Input: dimensioned drawing with shaded views. Units: mm. Origin: part minimum x, y, z. A direction names the side the tool comes from. Give positions to 0.01 mm unless a question says otherwise; leave off trailing zeros. Write each loop counter-clockwise with the first axis right and the second up, starting at its lowest first coordinate (ties: lowest second). Pieces come first, ordered by that corner, then holes.
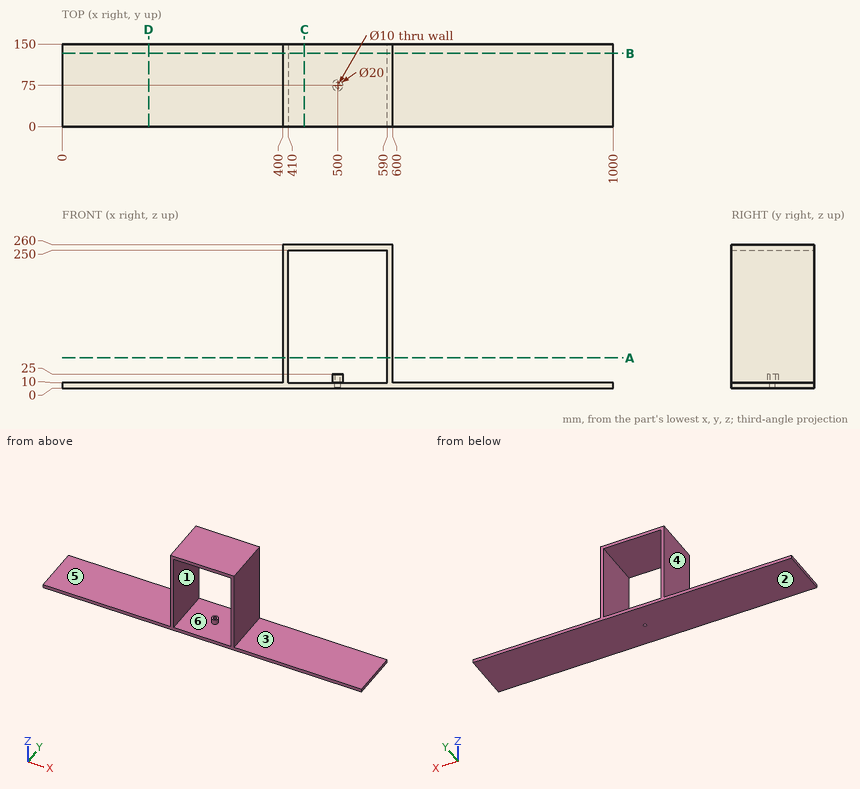
1. Cut plane A-A, the plane z = 54.5. Return the cut outline in (x, y), then the cut area to 3 significant figures.
2. Access query for the marked faces 1, 2 and 3. Directions: +Z, -Z, +X, -X, +Y, -Y. A direction counts if a zero-diameter tool reaches every point of the face in a straight line with its end or side. Return the directions, or none.
3. Cut plane C-C, the plane x = 439.5. Return the cut outline in (y, z), then the cut area to 3 significant figures.
4. Contact query for flat-ended pins moving along their axis: P1, Ø1, axis at y = 96, z = 135, coming from the -X side; P2, Ø1, axis at x = 167.5, y = 58, coming from the +Z side. Output: stop coordinate, or through.
5. Mould query, pull axis Z, two halves, no side actions, for the marked faces 4, 5 and 6. Classes: +Z half, -Z half, draft (parallel to the pull), parting line (faces both ways), or undercut.
6. Line query: L1, parallel to X at y = 75, z = 184.5; L2, parallel to Z at x = 449.5, y = 117; L3, parallel to Y at x = 500, z = 3. Output: solid intervals per line, ascending.
7. Cut plane D-D, the plane x = 157. Return the cut outline in (y, z), then the cut area to 3 significant figures.
8. Cut plane B-B, the plane y = 133. Return the cut outline in (x, z), then the cut area to 3 significant figures.
Response values:
1. outline: (400, 0) - (410, 0) - (410, 150) - (400, 150) - close; (590, 0) - (600, 0) - (600, 150) - (590, 150) - close
1. area: 3,000 mm2
2. face 1: +Y, -Y
2. face 2: -Z, +X, -X, +Y, -Y
2. face 3: +Z, +X, +Y, -Y
3. outline: (0, 0) - (150, 0) - (150, 10) - (0, 10) - close; (0, 250) - (150, 250) - (150, 260) - (0, 260) - close
3. area: 3,000 mm2
4. P1: stops at x = 400
4. P2: stops at z = 10
5. face 4: draft
5. face 5: +Z half
5. face 6: undercut
6. L1: x = 400 to 410, 590 to 600
6. L2: z = 0 to 10, 250 to 260
6. L3: y = 0 to 70, 80 to 150
7. outline: (0, 0) - (150, 0) - (150, 10) - (0, 10) - close
7. area: 1,500 mm2
8. outline: (0, 0) - (1000, 0) - (1000, 10) - (600, 10) - (600, 260) - (400, 260) - (400, 10) - (0, 10) - close; hole (410, 10) - (590, 10) - (590, 250) - (410, 250) - close
8. area: 16,800 mm2
